from build123d import *

# Parameters (mm, degrees)
BOSS_EXTRUDE1_DEPTH         = 12.446
F_1_4_0_25_DIAMETER_HOLE1_D = 6.35


with BuildPart() as part:
    # Sketch1 → Boss-Extrude1 (new body)
    with BuildSketch(Plane.XY):
        Polygon((-5.4737, 0), (5.4737, 0), (5.4737, -1.9177), (3.048, -4.3434), (-3.048, -4.3434), (-5.4737, -1.9177), align=None)
    extrude(amount=BOSS_EXTRUDE1_DEPTH)

    # 1/4 (0.25) Diameter Hole1 (through all)
    with Locations(Plane(origin=(0, 0, 0), x_dir=(1, 0, 0), z_dir=(0, 1, 0))):
        with Locations((0, -6.223)):
            Hole(F_1_4_0_25_DIAMETER_HOLE1_D / 2)


solid = part.part
Source: CAD feature listing. Evaluate the final solid. Frame: model axes, mm. Coordinates: 2 decimals unless noted, no trailing zeros. Order: outer loops, then holes, each group sorted by start corner. A loop starts at its lowest first (then second) coordinate and runs counter-clockwise, first axis right, second up. Notation, with made-up numbers: M 57.5,42 L 86.5,42 A21 cw 86.5,66 Z; hole C 16,24 d9. An arc over 180 degrees is marked long. Write each question's results on one line, items separated by ' | '. Start each with the question number.
1. Section B-B, the plane z = 9. Return the cut outline in (x, y).
2. Pin query (flat end, axial travel): pin 1 (5.5 mm diameter, centred on x = 0, z = 6.223, fed in from -Y). Return the tip coordinate at first contact, or that it passes through.
3. Material intervals for L1, parallel to Z at x = 0, y = -2.95; L2, parallel to X at y = -1.25, z = 5; L3, parallel to X at y = -3.2, z = 7.5, sorted ascending.
4. Draft query along X for faces 1 (the face through (0, -4.343, 2)), 2 (the face through (4.28, -3.11, 6.14)), 3 (the face through (-1.465, -2.202, 9.04)). Return one class per face: +X half, -X half, draft (parallel to the pull), parting line (faces both ways), or undercut.
5. Section C-C, the plane y = -0.3. Return the cut outline in (x, z) (3 decimals), then the cut area to 3 significant figures.
6. Section A-A, the plane x = 0. Return the cut outline in (y, z).
7. Section D-D, the plane z = 2.5. Return the cut outline in (x, y).
Solution:
1) outline: M -5.47,-1.92 L -3.05,-4.34 L -1.54,-4.34 L -1.54,0 L -5.47,0 Z; M 1.54,-4.34 L 3.05,-4.34 L 5.47,-1.92 L 5.47,0 L 1.54,0 Z
2) pin 1: through
3) L1: 0 to 3.05, 9.4 to 12.45 | L2: -5.47 to -2.93, 2.93 to 5.47 | L3: -4.19 to -2.91, 2.91 to 4.19
4) face 1: draft | face 2: +X half | face 3: undercut
5) outline: M -5.474,0 L 5.474,0 L 5.474,12.446 L -5.474,12.446 Z; hole C 0,6.223 d6.35 | area: 105 mm²
6) outline: M -4.34,0 L 0,0 L 0,3.05 L -4.34,3.05 Z; M -4.34,9.4 L 0,9.4 L 0,12.45 L -4.34,12.45 Z
7) outline: M -5.47,-1.92 L -3.05,-4.34 L 3.05,-4.34 L 5.47,-1.92 L 5.47,0 L -5.47,0 Z
